Geometry: final body of the model. Coordinates: model frame, mm. A direction names the side the tool comes from. Give positions to 0.01 mm unless a question says otherwise; leave off trailing zeros. Write each loop counter-clockwise with the first axis right and the second up, starting at its lowest first coordinate (ties: lowest second). Pieces come first, ordered by that corner, then holes.
Q1. Section A-A (x = 0). Return the cut outline in (y, z).
Q2. Pin query (flat end, axial travel): pin 1 Ø1 at (x, y) = (-1.5, -0.5) entering from -Z. Return the tip coordinate at first contact, or that it passes through.
Q3. Section B-B (y = 0). Return the cut outline in (x, z).
Q4. Line query: line 1 (Y direction, x = 0, z = 65.5); line 2 (Z direction, x = 0, y = -4.4); line 3 (Z direction, x = -3, y = -0.5). Output: solid intervals per line, ascending.
Q5. Section C-C (z = 81). Return the cut outline in (x, y).
Q6. Mould query, pull axis Y, two halves, no side actions, for faces 1 (the flat face through (-5, 0, 60)), 2 (the flat face through (0, 5, 60)), 3 (the cylindrical face through (0.521, 3.966, 59.16)). Classes: +Y half, -Y half, draft (parallel to the pull), parting line (faces both ways), or undercut.
Q7. Reachability of faces 4 (the flat face through (0, 0, 120)), 5 (the cylindrical face through (1.91, -4.41, 6.83)), 6 (the flat face through (0, 0, 122)) from +Z, -Z, +X, -X, +Y, -Y: full face, straight path, thin tool, end or side. Return the list, or none.
from build123d import *

# Parameters (mm, degrees)
SKETCH_1_W          = 10
SKETCH_1_H          = 10
EXTRUDE_1_DEPTH     = 122
SKETCH_2_R          = 4
CUT_EXTRUDE_1_DEPTH = 120
SKETCH_3_R          = 2
CUT_EXTRUDE_2_DEPTH = 2


with BuildPart() as part:
    # 草图1 → 凸台-拉伸1 (new body)
    with BuildSketch(Plane.XY):
        Rectangle(SKETCH_1_W, SKETCH_1_H)
    extrude(amount=EXTRUDE_1_DEPTH)

    # 草图2 → 切除-拉伸1 (cut)
    with BuildSketch(Plane(origin=(0, 0, 0), x_dir=(-1, 0, 0), z_dir=(0, 0, -1))):
        Circle(SKETCH_2_R)
    extrude(amount=-CUT_EXTRUDE_1_DEPTH, mode=Mode.SUBTRACT)

    # 草图3 → 切除-拉伸2 (cut)
    with BuildSketch(Plane.XZ.offset(5)):
        with Locations((0, 6.231427265)):
            Circle(SKETCH_3_R)
    extrude(amount=-CUT_EXTRUDE_2_DEPTH, mode=Mode.SUBTRACT)


solid = part.part
Computed:
1. outline: (-5, 0) - (-4, 0) - (-4, 4.23) - (-5, 4.23) - close; (-5, 8.23) - (-4, 8.23) - (-4, 120) - (4, 120) - (4, 0) - (5, 0) - (5, 122) - (-5, 122) - close
2. pin 1: stops at z = 120
3. outline: (-5, 0) - (-4, 0) - (-4, 120) - (4, 120) - (4, 0) - (5, 0) - (5, 122) - (-5, 122) - close
4. line 1: y = -5 to -4, 4 to 5
4. line 2: z = 0 to 4.23, 8.23 to 122
4. line 3: z = 120 to 122
5. outline: (-5, -5) - (5, -5) - (5, 5) - (-5, 5) - close; hole circle Ø8 at (0, 0)
6. face 1: draft
6. face 2: +Y half
6. face 3: undercut
7. face 4: -Z
7. face 5: -Y
7. face 6: +Z, +X, -X, +Y, -Y
